Part model, mm, in its own coordinate system. A direction names the side the tool comes from. Round coordinates to 2 decimals unless told otherwise and drop trailing zeros. Loops run counter-clockwise (first coordinate to the right, second up) from the corner with the lowest first, then second, coordinate; pieces in that order, holes last. Notation, with made-up numbers: (87, 27.25) -> (122, 27.25) arc R24 cw to (122, 54.25) -> close; hole circle Ø11 at (18, 54.5). An arc over 180 degrees is marked (long way). Use a Markdown table: item, result. Add a question column.
Item 1: Which spindle directions (+Z, -Z, +X, -X, +Y, -Y) get a long thin tool onto all of the face, cutting with end or side? Do faces 5 (the face through (2.67, 58.14, -5.53)), 6 (the face through (1, 3, 21)), 7 (the face through (0, 38, 0)), 8 (the face through (-2.493, 60.687, -5.596)). Say none if no direction does.
Item 2: Cut at B-B, the plane x = 12. List the corners of the cut face in (y, z).
Item 3: Cut at D-D, the plane z = 5. List the corners of the cut face in (x, y).
Item 4: Probe line 1 (X direction, y = 52, z = 0); line 2 (Y direction, x = -43.5, z = -40.5); line 3 (Y direction, x = -27.5, z = -32). List the from-to ranges inside material, lowest first. Write a range as [from, to].
Item 5: Cut at A-A, the plane y = 6.5. List the corners of the cut face in (x, z).
Item 6: Two-plate mould, pull along X, no slides. Class faces 1 (the face through (-27.627, 18.776, -28.881)), 2 (the face through (0, 13, 0)), 3 (the face through (-0.788, 60.463, -6.701)), 4 (the face through (-1, 68, 2)): pulls with the +X half, pulls with the -X half, needs draft (parallel to the pull), parting line crosses it, or undercut.
Item 7: Flat gauge pins, fed straight in: pin 1 (1.3 mm diameter, centred on x = 1.5, z = -5, fed in from +Y); pin 2 (3 mm diameter, centred on x = 55, z = 15, fed in from +Y); pin 3 (2.5 mm diameter, centred on x = 0.5, z = -0.5, fed in from +Y). Where does each tip first touch, or does it go through?
Item 8: Cut at C-C, the plane z = -59.5. List the corners of the cut face in (x, y), plus the area to 3 significant figures.
```python
from build123d import *
from build123d.topology import SkipClean

# Parameters (mm, degrees)
SKETCH3_R               = 70.5
BOSS_EXTRUDE2_DEPTH     = 38
SKETCH4_R               = 22.5
CUT_EXTRUDE1_DEPTH      = 89
CUT_EXTRUDE2_START      = -35
CUT_EXTRUDE2_DEPTH      = 35
SKETCH8_R               = 10
BOSS_EXTRUDE3_DEPTH     = 65
CUT_EXTRUDE4_DEPTH      = 30
CUT_EXTRUDE5_START      = -3
CUT_EXTRUDE5_DEPTH      = 3
CUT_EXTRUDE6_START      = -10
CUT_EXTRUDE6_DEPTH      = 10
CUT_EXTRUDE7_DEPTH      = 20
CUT_EXTRUDE9_DEPTH      = 12
CUT_EXTRUDE9_DEPTH_BACK = 12
SKETCH14_R              = 1.55
CUT_EXTRUDE10_DEPTH     = 7
SKETCH16_R              = 3.05
CUT_EXTRUDE11_DEPTH     = 7


with BuildPart() as part:
    # Sketch3 → Boss-Extrude2 (new body)
    with BuildSketch(Plane(origin=(0, 0, 0), x_dir=(1, 0, 0), z_dir=(0, 1, 0))):
        with Locations(Location((0, 0, 0), (0, 0, 270))):
            Circle(SKETCH3_R)
    extrude(amount=BOSS_EXTRUDE2_DEPTH)

    # Sketch4 → Cut-Extrude1 (cut)
    with BuildSketch(Plane(origin=(0, 38, 0), x_dir=(1, 0, 0), z_dir=(0, 1, 0))):
        with Locations(Location((0, 40, 0), (0, 0, 270))):
            Circle(SKETCH4_R)
        with BuildLine():
            Line((1.445129752, -2.04), (-1.445129752, -2.04))
            ThreePointArc((-1.445129752, -2.04), (0, 2.5), (1.445129752, -2.04))
        make_face()
    extrude(amount=-CUT_EXTRUDE1_DEPTH, mode=Mode.SUBTRACT)

    # Sketch6 → Cut-Extrude2 (cut)
    with BuildSketch(Plane(origin=(0, 38, 0), x_dir=(1, 0, 0), z_dir=(0, 1, 0)).offset(CUT_EXTRUDE2_START)):
        with BuildLine():
            Line((-45.196231291, 54.106845011), (-0.557111742, -9.984469265))
            Line((-0.557111742, -9.984469265), (49.803768709, 49.898242679))
            ThreePointArc((49.803768709, 49.898242679), (-3.120165646, -70.430920527), (-45.196231291, 54.106845011))
        make_face()
    extrude(amount=CUT_EXTRUDE2_DEPTH, mode=Mode.SUBTRACT)

    # Sketch8 → Boss-Extrude3 (add)
    with BuildSketch(Plane(origin=(0, 3, 0), x_dir=(1, 0, 0), z_dir=(0, 1, 0))):
        with Locations(Location((0, 0, 0), (0, 0, 162.907512523))):
            Circle(SKETCH8_R)
    extrude(amount=BOSS_EXTRUDE3_DEPTH)

    # Sketch10 → Cut-Extrude4 (cut)
    with BuildSketch(Plane(origin=(0, 68, 0), x_dir=(1, 0, 0), z_dir=(0, 1, 0))):
        with BuildLine():
            Line((-1.99989737, -1.516743389), (0.826538727, -2.370007117))
            ThreePointArc((0.826538727, -2.370007117), (0.725401526, 2.402892554), (-1.99989737, -1.516743389))
        make_face()
    extrude(amount=-CUT_EXTRUDE4_DEPTH, mode=Mode.SUBTRACT)

    # Sketch11 → Cut-Extrude5 (cut)
    with SkipClean():  # the faces are left unmerged after this step: merging them gives an invalid solid
        with BuildSketch(Plane(origin=(0, 38, 0), x_dir=(1, 0, 0), z_dir=(0, 1, 0)).offset(CUT_EXTRUDE5_START)):
            with BuildLine():
                Line((-45.196231291, 54.106845011), (-9.558315606, 2.939150008))
                ThreePointArc((-9.558315606, 2.939150008), (0.351258268, 9.993828977), (9.741081782, 2.260824122))
                Line((9.741081782, 2.260824122), (49.803768709, 49.898242679))
                ThreePointArc((49.803768709, 49.898242679), (3.120165646, 70.430920527), (-45.196231291, 54.106845011))
            make_face()
        extrude(amount=CUT_EXTRUDE5_DEPTH, mode=Mode.SUBTRACT)

    # Sketch12 → Cut-Extrude6 (cut)
    with SkipClean():  # the faces are left unmerged after this step: merging them gives an invalid solid
        with BuildSketch(Plane.XZ.offset(-3).offset(CUT_EXTRUDE6_START)):
            with BuildLine():
                Line((-1.445129752, 2.04), (1.445129752, 2.04))
                ThreePointArc((1.445129752, 2.04), (0, -2.5), (-1.445129752, 2.04))
            make_face()
        extrude(amount=CUT_EXTRUDE6_DEPTH, mode=Mode.SUBTRACT)

    # Sketch13 → Cut-Extrude7 (cut)
    with SkipClean():  # the faces are left unmerged after this step: merging them gives an invalid solid
        with BuildSketch(Plane(origin=(0, 68, 0), x_dir=(1, 0, 0), z_dir=(0, 1, 0))):
            Polygon((-0.496518118, 2.460400325), (1.674568679, 1.86973788), (3.774701815, 9.5891576), (1.603615019, 10.179820045), align=None)
        extrude(amount=-CUT_EXTRUDE7_DEPTH, mode=Mode.SUBTRACT)

    # Sketch14 → Cut-Extrude9 (cut, two sides: drawn at the far end of the back side and taken through both)
    with SkipClean():  # the faces are left unmerged after this step: merging them gives an invalid solid
        with BuildSketch(Plane(origin=(-1.085543398, 0, -0.295331222), x_dir=(0.2625166420985644, 0, -0.9649274649533479), z_dir=(0.9649274649533479, 0, 0.2625166420985644)).offset(-CUT_EXTRUDE9_DEPTH_BACK)):
            with Locations(Location((6.057727773, 62, 0), (0, 0, 180))):
                Circle(SKETCH14_R)
        extrude(amount=CUT_EXTRUDE9_DEPTH + CUT_EXTRUDE9_DEPTH_BACK, mode=Mode.SUBTRACT)

    # Sketch15 → Cut-Extrude10 (cut)
    with SkipClean():  # the faces are left unmerged after this step: merging them gives an invalid solid
        with BuildSketch(Plane(origin=(10.493586181, 0, 2.854868483), x_dir=(0.2625166420985644, 0, -0.9649274649533479), z_dir=(0.9649274649533479, 0, 0.2625166420985644))):
            Polygon((9.107727773, 62), (7.582727773, 64.641377482), (4.532727773, 64.641377482), (3.007727773, 62), (4.532727773, 59.358622518), (7.582727773, 59.358622518), align=None)
        extrude(amount=-CUT_EXTRUDE10_DEPTH, mode=Mode.SUBTRACT)

    # Sketch16 → Cut-Extrude11 (cut)
    with SkipClean():  # the faces are left unmerged after this step: merging them gives an invalid solid
        with BuildSketch(Plane(origin=(-10.493586181, 0, -2.854868483), x_dir=(-0.26251664209856435, 0, 0.9649274649533478), z_dir=(-0.9649274649533478, 0, -0.26251664209856435))):
            with Locations((-6.057727773, 62)):
                Circle(SKETCH16_R)
        extrude(amount=-CUT_EXTRUDE11_DEPTH, mode=Mode.SUBTRACT)


solid = part.part
```
A:
| question | item | result |
|---|---|---|
| 1 | face 5 | -Z, +Y |
| 1 | face 6 | +Z, +Y |
| 1 | face 7 | +Y |
| 1 | face 8 | none |
| 2 | outline | (0, -69.47) -> (35, -69.47) -> (35, -59.03) -> (0, -59.03) -> close; (0, -20.97) -> (35, -20.97) -> (35, -4.95) -> (3, -4.95) -> (3, 69.47) -> (0, 69.47) -> close |
| 3 | outline | (-70.32, 0) -> (70.32, 0) -> (70.32, 3) -> (8.66, 3) -> (8.66, 68) -> (-8.66, 68) -> (-8.66, 3) -> (-70.32, 3) -> close |
| 4 | line 1 | x = [-10, -2.51], [2.51, 10] |
| 4 | line 2 | y = [0, 3] |
| 4 | line 3 | y = [0, 35] |
| 5 | outline | (-45.2, -54.11) arc R70.5 ccw to (49.8, -49.9) -> (9.74, -2.26) arc R10 ccw (long way) to (-9.56, -2.94) -> close; hole circle Ø45 at (0, -40); hole (-1.45, 2.04) arc R2.5 ccw (long way) to (1.45, 2.04) -> close |
| 6 | face 1 | pulls with the -X half |
| 6 | face 2 | undercut |
| 6 | face 3 | undercut |
| 6 | face 4 | needs draft |
| 7 | pin 1 | stops at y = 48 |
| 7 | pin 2 | stops at y = 3 |
| 7 | pin 3 | stops at y = 38 |
| 8 | outline | (-37.82, 0) -> (-11.22, 0) -> (-11.22, 35) -> (-37.82, 35) -> close; (11.22, 0) -> (37.82, 0) -> (37.82, 35) -> (11.22, 35) -> close |
| 8 | area | 1,860 mm^2 |
